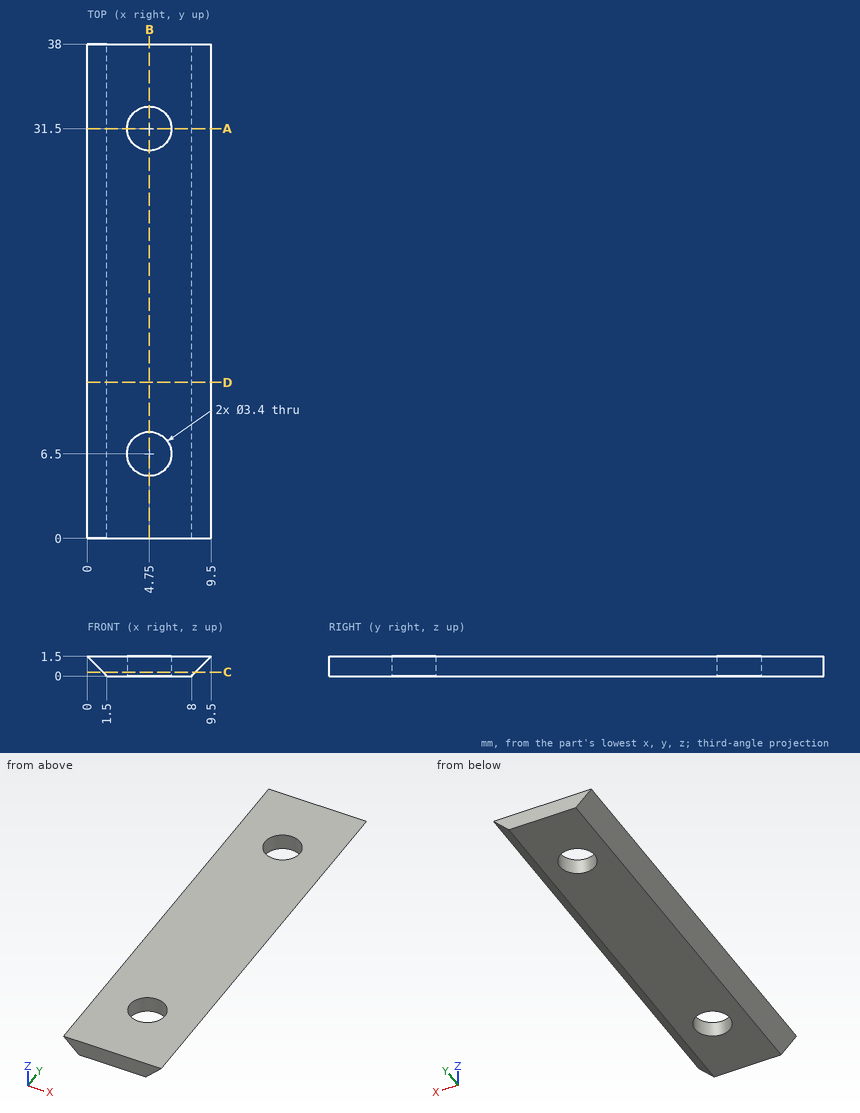
Study the drawing (mm; zero at the part's minimum x, y, z) and answer. Coordinates: 2 decimals unless noted, no trailing zeros. Write each loop counter-clockwise with the first axis right and the second up, starting at its lowest first coordinate (ties: lowest second). Pieces come first, ordered by that corner, then holes. Notation, with made-up numbers: (66.25, 56) - (102.25, 56) arc R15 ccw to (102.25, 64) - close; hole circle Ø3 at (-14, 58.25). An arc over 180 degrees is marked (long way). One line per question, with ' | ' between items.
1) Find section A-A, the plane y = 31.5. Determine the outline of the cut face in (x, z), and give its area (3 significant figures).
Checks:
outline: (0, 1.5) - (1.5, 0) - (3.05, 0) - (3.05, 1.5) - close; (6.45, 0) - (8, 0) - (9.5, 1.5) - (6.45, 1.5) - close | area: 6.90 mm2
2) Find section B-B, the plane x = 4.75. Determine the outline of the cut face in (y, z), and give its area (3 significant figures).
Checks:
outline: (0, 0) - (4.8, 0) - (4.8, 1.5) - (0, 1.5) - close; (8.2, 0) - (29.8, 0) - (29.8, 1.5) - (8.2, 1.5) - close; (33.2, 0) - (38, 0) - (38, 1.5) - (33.2, 1.5) - close | area: 46.8 mm2
3) Find section D-D, the plane y = 12. Determine the outline of the cut face in (x, z).
Checks:
outline: (0, 1.5) - (1.5, 0) - (8, 0) - (9.5, 1.5) - close
4) Consider probe 1 along Y at (x, z) = (4.75, 0.6); probe 2 along Y at (x, z) = (4, 0.8); probe 3 along X at (y, z) = (6.5, 0.8). Determine where each line is inside the solid, lowest interval first. Write a range as [from, to].
Checks:
probe 1: [0, 4.8], [8.2, 29.8], [33.2, 38] | probe 2: [0, 4.97], [8.03, 29.97], [33.03, 38] | probe 3: [0.7, 3.05], [6.45, 8.8]
5) Find section C-C, the plane z = 0.3. Determine the outline of the cut face in (x, y), and give its area (3 significant figures).
Checks:
outline: (1.2, 0) - (8.3, 0) - (8.3, 38) - (1.2, 38) - close; hole circle Ø3.4 at (4.75, 6.5); hole circle Ø3.4 at (4.75, 31.5) | area: 252 mm2
